The listing builds one solid part. Answer for the finished solid, in the listing's coordinates (mm). A direction names the side the tool comes from. Coordinates: 2 decimals unless noted, no trailing zeros. Write each loop counter-clockwise with the first axis right and the second up, starting at its lowest first coordinate (ties: lowest second). Pieces come first, ordered by that corner, then holes.
(1) The part is cut by section A-A on y = 0. Determine the outline of the cut face in (x, z), plus the area to 3 significant figures.
(2) Given P1, Ø13.5, axis at x = -5, z = 28, coming from the +Y side; P2, Ø12, axis at y = 6, z = 14, coming from the +X side; P3, Ø2, axis at x = -18.5, z = 16.5, coming from the +Y side; P4, Ø4.5, axis at y = 0, z = 34.44, coming from the -X side, each flat-ended and moving along its own axis, determine where each tip first touches the part or whether it passes through.
(3) For a pull along Y with two mould halves and no side action, classify faces 1 (the flat face through (-26, -12, 0)), 2 (the cylindrical face through (-27.46, 0.08, 6.58)), 3 (the flat face through (-15, -39.974, 20)) as +Y half, -Y half, draft (parallel to the pull), parting line (faces both ways), or undercut.
(4) The part is cut by section B-B on z = 28. Determine the outline of the cut face in (x, y).
(5) The part is cut by section C-C on x = -7.75. Determine the outline of the cut face in (y, z).
(6) Which of the six approach directions +Z, -Z, +X, -X, +Y, -Y give full straight-line access (tool end or side, diameter ignored) to faces 4 (the cylindrical face through (-27.46, 22.37, 5.06)), 5 (the flat face through (-8, -34.974, 20))?
(7) The part is cut by section D-D on y = -29.5. Determine the outline of the cut face in (x, z), plus the area to 3 significant figures.
(8) Straight lines are drawn through the part: line 1 (X direction, y = -21.5, z = 7.5); line 2 (Y direction, x = -2, z = 33); line 3 (X direction, y = -32.5, z = 31.5). For each, find the intervals that lie inside material, in ascending order.
from build123d import *

# Parameters (mm, degrees)
RESSALTO_EXTRUS_O1_DEPTH                   = 40
BROCA_DE_ROSQUEAR_PARA_HELICOIDE_M31_D     = 3.5
BROCA_DE_ROSQUEAR_PARA_HELICOIDE_M31_DEPTH = 10
BROCA_DE_ROSQUEAR_PARA_HELICOIDE_M31_TIP   = 1.051506083
BROCA_DE_ROSQUEAR_PARA_HELICOIDE_M32_D     = 3.5
BROCA_DE_ROSQUEAR_PARA_HELICOIDE_M32_DEPTH = 10
BROCA_DE_ROSQUEAR_PARA_HELICOIDE_M32_TIP   = 1.051506083
FILETE1_R                                  = 8


with BuildPart() as part:
    # Esboço1 → Ressalto-extrusão1 (new body)
    with BuildSketch(Plane.XY):
        Polygon((-30, 40.02617801), (-30, -39.97382199), (0, -39.97382199), (0, -34.97382199), (-25, -34.97382199), (-25, 40.02617801), align=None)
    extrude(amount=RESSALTO_EXTRUS_O1_DEPTH)

    # Broca de rosquear para helicoide M31
    with Locations(Plane(origin=(0, -34.97382199, 0), x_dir=(1, 0, 0), z_dir=(0, 1, 0))):
        with Locations((-13.529029312, -32.612904954), (-13.529029312, -10.11076891)):
            Hole(BROCA_DE_ROSQUEAR_PARA_HELICOIDE_M31_D / 2, depth=BROCA_DE_ROSQUEAR_PARA_HELICOIDE_M31_DEPTH)
            with Locations((0, 0, -(BROCA_DE_ROSQUEAR_PARA_HELICOIDE_M31_DEPTH + BROCA_DE_ROSQUEAR_PARA_HELICOIDE_M31_TIP / 2))):  # 118° drill point
                Cone(0, BROCA_DE_ROSQUEAR_PARA_HELICOIDE_M31_D / 2, BROCA_DE_ROSQUEAR_PARA_HELICOIDE_M31_TIP, mode=Mode.SUBTRACT)

    # Broca de rosquear para helicoide M32
    with Locations(Plane.ZY.offset(30)):
        with Locations((4.832044367, 20.635096837), (34.443923193, 20.635096837), (34.443923193, 0), (4.832044367, 0)):
            Hole(BROCA_DE_ROSQUEAR_PARA_HELICOIDE_M32_D / 2, depth=BROCA_DE_ROSQUEAR_PARA_HELICOIDE_M32_DEPTH)
            with Locations((0, 0, -(BROCA_DE_ROSQUEAR_PARA_HELICOIDE_M32_DEPTH + BROCA_DE_ROSQUEAR_PARA_HELICOIDE_M32_TIP / 2))):  # 118° drill point
                Cone(0, BROCA_DE_ROSQUEAR_PARA_HELICOIDE_M32_D / 2, BROCA_DE_ROSQUEAR_PARA_HELICOIDE_M32_TIP, mode=Mode.SUBTRACT)

    # Filete1
    filete1_edges = [part.edges().sort_by_distance(p)[0] for p in [
        (-25, -34.97382199, 20),
    ]]
    fillet(filete1_edges, radius=FILETE1_R)


solid = part.part
Model answer:
1. outline: (-30, 0) - (-25, 0) - (-25, 3.08) - (-30, 3.08) - close; (-30, 6.58) - (-25, 6.58) - (-25, 32.69) - (-30, 32.69) - close; (-30, 36.19) - (-25, 36.19) - (-25, 40) - (-30, 40) - close
1. area: 165 mm2
2. P1: stops at y = -34.97
2. P2: stops at x = -25
2. P3: stops at y = -34.57
2. P4: stops at x = -30
3. face 1: draft
3. face 2: undercut
3. face 3: -Y half
4. outline: (-30, -39.97) - (0, -39.97) - (0, -34.97) - (-17, -34.97) arc R8 cw to (-25, -26.97) - (-25, 40.03) - (-30, 40.03) - close
5. outline: (-39.97, 0) - (-34.97, 0) - (-34.97, 40) - (-39.97, 40) - close
6. face 4: +X, -X
6. face 5: +Z, -Z, +X, +Y
7. outline: (-30, 0) - (-24.59, 0) - (-24.59, 40) - (-30, 40) - close
7. area: 216 mm2
8. line 1: x = -30 to -25
8. line 2: y = -39.97 to -34.97
8. line 3: x = -30 to -22.78
